from build123d import *

# Parameters (mm, degrees)
SKETCH_1_R      = 8.4
EXTRUDE_1_DEPTH = 15.9
SKETCH_2_R      = 11.75
EXTRUDE_2_DEPTH = 2.5
SKETCH_3_R      = 3.825
EXTRUDE_3_DEPTH = 6.5
CHAMFER_1_SIZE  = 1
CHAMFER_2_SIZE  = 0.1


with BuildPart() as part:
    # Эскиз1 → Бобышка-Вытянуть1 (new body)
    with BuildSketch(Plane(origin=(0, 0, 0), x_dir=(1, 0, 0), z_dir=(0, 1, 0))):
        with Locations(Location((0, 0, 0), (0, 0, 270))):
            Circle(SKETCH_1_R)
    extrude(amount=EXTRUDE_1_DEPTH)

    # Эскиз2 → Бобышка-Вытянуть2 (add)
    with BuildSketch(Plane(origin=(0, 15.9, 0), x_dir=(1, 0, 0), z_dir=(0, 1, 0))):
        with Locations(Location((0, 0, 0), (0, 0, 270))):
            Circle(SKETCH_2_R)
    extrude(amount=EXTRUDE_2_DEPTH)

    # Эскиз3 → Бобышка-Вытянуть3 (add)
    with BuildSketch(Plane(origin=(0, 18.4, 0), x_dir=(1, 0, 0), z_dir=(0, 1, 0))):
        with Locations(Location((0, 0, 0), (0, 0, 90))):
            Circle(SKETCH_3_R)
    extrude(amount=EXTRUDE_3_DEPTH)

    # Фаска1
    chamfer_1_edges = [part.edges().sort_by_distance(p)[0] for p in [
        (0, 0, -8.4),
        (0, 18.4, -11.75),
    ]]
    chamfer(chamfer_1_edges, length=CHAMFER_1_SIZE)

    # Фаска2
    chamfer_2_edges = [part.edges().sort_by_distance(p)[0] for p in [
        (0, 24.9, 3.825),
        (0, 18.4, 3.825),
    ]]
    chamfer(chamfer_2_edges, length=CHAMFER_2_SIZE)


solid = part.part
Design review of the part built by this model. Coordinates are the model's own, in mm. A direction names the side the tool comes from. Coordinates: 2 decimals unless noted, no trailing zeros. Write each loop counter-clockwise with the first axis right and the second up, starting at its lowest first coordinate (ties: lowest second). Pieces come first, ordered by that corner, then holes. Notation, with made-up numbers: (50.25, 71) - (102.25, 71) arc R10 ccw to (102.25, 79) - close; hole circle Ø7 at (82, 2.5). An arc over 180 degrees is marked (long way). One line per item, written item: value.
1) To check wall thickness, follow probe 1 along Y at (x, z) = (-8.5, -2.5); probe 2 along Y at (x, z) = (5, 1.5); probe 3 along Z at (x, y) = (2.25, 2.75). State the ranges of each line that lie inside material, in increasing order.
Answer sheet:
probe 1: y = 15.9 to 18.4
probe 2: y = 0 to 18.4
probe 3: z = -8.09 to 8.09
2) Add section C-C (y = 20.25). State the section outline as (x, z) points (3 decimals).
Answer sheet:
outline: circle Ø7.65 at (0, 0)
3) Add section A-A (z = 0). State the section outline as (x, y) points (3 decimals), plus the area to 3 significant figures.
Answer sheet:
outline: (-11.75, 15.9) - (-8.4, 15.9) - (-8.4, 1) - (-7.4, 0) - (7.4, 0) - (8.4, 1) - (8.4, 15.9) - (11.75, 15.9) - (11.75, 17.4) - (10.75, 18.4) - (3.925, 18.4) - (3.825, 18.5) - (3.825, 24.8) - (3.725, 24.9) - (-3.725, 24.9) - (-3.825, 24.8) - (-3.825, 18.5) - (-3.925, 18.4) - (-10.75, 18.4) - (-11.75, 17.4) - close
area: 374 mm2
4) For faces 1 (the face through (0, 18.4, 5)), 2 (the face through (0, 24.9, 0)), 3 (the face through (2.523, 8.346, 8.012)), list the 3-axis set-ups (+Z, -Z, +X, -X, +Y, -Y) from which the entire face can be reached by the end or side of a thin tool; tool diameter is ignored.
Answer sheet:
face 1: +Y
face 2: +Z, -Z, +X, -X, +Y
face 3: -Y
5) Insertion check: pin 1 (1.5 mm diameter, centred on y = 14.5, z = -6.5, fed in from -X); pin 2 (1 mm diameter, centred on x = -9, y = 18.5, fed in from -Z); pin 3 (5 mm diameter, centred on x = -4, y = 7.5, fed in from -Z) (3 decimals). Each pin has a flat end and moves straight along its axis. Give the tip position at first contact, or say it passes through.
Answer sheet:
pin 1: stops at x = -6.12
pin 2: stops at z = -6.81
pin 3: stops at z = -8.265
6) Add section B-B (x = 0). State the section outline as (y, z) points (3 decimals), plus the area to 3 significant figures.
Answer sheet:
outline: (0, -7.4) - (1, -8.4) - (15.9, -8.4) - (15.9, -11.75) - (17.4, -11.75) - (18.4, -10.75) - (18.4, -3.925) - (18.5, -3.825) - (24.8, -3.825) - (24.9, -3.725) - (24.9, 3.725) - (24.8, 3.825) - (18.5, 3.825) - (18.4, 3.925) - (18.4, 10.75) - (17.4, 11.75) - (15.9, 11.75) - (15.9, 8.4) - (1, 8.4) - (0, 7.4) - close
area: 374 mm2
7) Add section D-D (y = 12). State the section outline as (x, z) points.
Answer sheet:
outline: circle Ø16.8 at (0, 0)
